from build123d import *

# Parameters (mm, degrees)
F0_R     = 2.65
F1_DEPTH = 10
F2_W     = 9.2
F2_H     = 10
F2_H_2   = 3
F3_DEPTH = 4
F4_W     = 17.5
F4_H     = 10
F4_H_2   = 3
F5_DEPTH = 4


with BuildPart() as f1:
    # F0 (on Top) → F1 (new body)
    with BuildSketch(Plane.XY):
        with BuildLine():
            Line((-18, 7.8823786229), (-18, -17.1176213771))
            Line((-18, -17.1176213771), (-0.5, -17.1176213771))
            Line((-0.5, -17.1176213771), (-0.5, -0.8176213771))
            ThreePointArc((-0.5, -0.8176213771), (4.15, 0.1823786229), (8.8, -0.8176213771))
            Line((8.8, -0.8176213771), (8.8, -17.1176213771))
            Line((8.8, -17.1176213771), (18, -17.1176213771))
            Line((18, -17.1176213771), (18, 7.8823786229))
            ThreePointArc((18, 7.8823786229), (0, 16.8823786229), (-18, 7.8823786229))
        make_face()
        with Locations((-9, 4.3823786229)):
            Circle(F0_R, mode=Mode.SUBTRACT)
        with Locations((4.15, 7.8823786229)):
            Circle(F0_R, mode=Mode.SUBTRACT)
    extrude(amount=F1_DEPTH)

    # F2 (on face) → F3 (join)
    with BuildSketch(Plane.XZ.offset(17.1176213771)):
        with Locations((13.4, 5)):
            Rectangle(F2_W, F2_H)
        with Locations((13.4, 11.5)):
            Rectangle(F2_W, F2_H_2)
    extrude(amount=F3_DEPTH)

    # F4 (on face) → F5 (join, through all)
    with BuildSketch(Plane.XZ.offset(17.1176213771)):
        with Locations((-9.25, 5)):
            Rectangle(F4_W, F4_H)
        with Locations((-9.25, 11.5)):
            Rectangle(F4_W, F4_H_2)
    extrude(amount=F5_DEPTH)


solid = f1.part
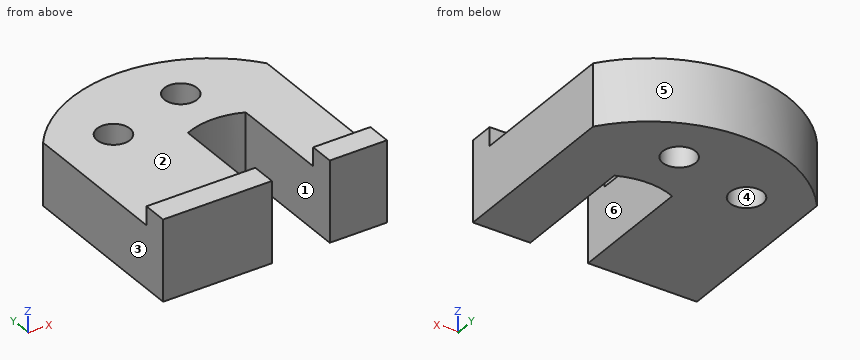
The listing builds one solid part. Answer for the finished solid, in the listing's coordinates (mm). Face numbers are marked on the shaded views. A direction names the side the tool comes from. Give positions to 0.01 mm unless a question says otherwise; leave off trailing zeros. Order: outer loops, then holes, each group sorted by start corner. A loop starts at its lowest first (then second) coordinate and runs counter-clockwise, first axis right, second up. Notation, with made-up numbers: (82.25, 87.5) -> (98.25, 87.5) arc R23 ccw to (98.25, 102.5) -> close; hole circle Ø10 at (81.25, 0.25). An arc over 180 degrees is marked (long way). Put each result on its own line as item: value.
Item 1: Given P1, Ø2.5, axis at x = -12, z = 11, coming from the +Y side; P2, Ø10, axis at x = -9, y = 7.5, coming from the +Z side; P3, Ø1.5, axis at x = 15.5, z = 12, coming from the +Y side, each flat-ended and moving along its own axis, determine where each tip first touches the part or whether it passes through.
Established:
P1: stops at y = 13.87
P2: stops at z = 10
P3: stops at y = -17.12
Item 2: Straight lines are drawn through the part: line 1 (X direction, y = -8.5, z = 3.5); line 2 (Y direction, x = 4.15, z = 8); line 3 (Z direction, x = -7, y = -8). For each, find the intervals that lie inside material, in ascending order.
Established:
line 1: x = -18 to -0.5, 8.8 to 18
line 2: y = 0.18 to 5.23, 10.53 to 16.5
line 3: z = 0 to 10
Item 3: A cutting plane is placed at B-B on x = 4.15. Give the vertices of the cut face in (y, z).
Established:
outline: (0.18, 0) -> (5.23, 0) -> (5.23, 10) -> (0.18, 10) -> close; (10.53, 0) -> (16.5, 0) -> (16.5, 10) -> (10.53, 10) -> close
Item 4: For the marked faces 1, 2 and 3, determine the directions among +Z, -Z, +X, -X, +Y, -Y from which every point of the face is accessible in a straight line to the end or side of a thin tool.
Established:
face 1: +Z, -Z, -Y
face 2: +Z, +X, -X, +Y
face 3: +Z, -Z, -X, +Y, -Y
Item 5: For a pull along Y with two mould halves and no side action, classify the marked faces 4, 5 and 6 as released by +Y, released by -Y, zero draft, split by the parting line, or undercut.
Established:
face 4: undercut
face 5: released by +Y
face 6: zero draft
Item 6: A cutting plane is placed at D-D on x = -4.5. Give the vertices of the cut face in (y, z), plus the area to 3 significant figures.
Established:
outline: (-21.12, 0) -> (16.43, 0) -> (16.43, 10) -> (-17.12, 10) -> (-17.12, 13) -> (-21.12, 13) -> close
area: 387 mm^2
Item 7: A cutting plane is placed at A-A on y = -15. Give the vertices of the cut face in (x, z), plus the area to 3 significant figures.
Established:
outline: (-18, 0) -> (-0.5, 0) -> (-0.5, 10) -> (-18, 10) -> close; (8.8, 0) -> (18, 0) -> (18, 10) -> (8.8, 10) -> close
area: 267 mm^2
Item 8: A cutting plane is placed at C-C on z = 1. Give the vertices of the cut face in (x, y), plus the area to 3 significant figures.
Established:
outline: (-18, -21.12) -> (-0.5, -21.12) -> (-0.5, -0.82) arc R11.31 cw to (8.8, -0.82) -> (8.8, -21.12) -> (18, -21.12) -> (18, 7.88) arc R22.5 ccw to (-18, 7.88) -> close; hole circle Ø5.3 at (-9, 4.38); hole circle Ø5.3 at (4.15, 7.88)
area: 1,030 mm^2
